The figure shows three views and two pictorial views of one solid part (mm, origin at its lowest corner). Answer the questions. Round coordinates to 2 decimals unless told otherwise and drop trailing zeros. Order: outer loops, then holes, each group sorted by start corner. A loop starts at its lowest first (then second) coordinate and runs counter-clockwise, first axis right, second up. Notation, with made-up numbers: (52.5, 15) -> (59.5, 15) arc R26 ccw to (59.5, 45) -> close; hole circle Ø6 at (-25.75, 88.5). An arc over 180 degrees is marked (long way). Return JSON: item names as keys, results as strings. Group by question number.
(1) The part is cut by section A-A (x = 190.5). Determine the outline of the cut face in (y, z) (1 decimal).
(2) Consider line 1 (X direction, y = 2.15, z = 203.2); line 2 (Z direction, x = 190.5, y = 1); line 3 (Z direction, x = 30.48, y = 1.5). Determine where each line is inside the solid, lowest interval first. Write a range as [from, to].
(3) This flat-tipped pin is pushed along its axis until it touches: pin 1 (4 mm diameter, centred on x = 12.7, z = 50.8, fed in from +Y). Where does it stop, or does it pass through?
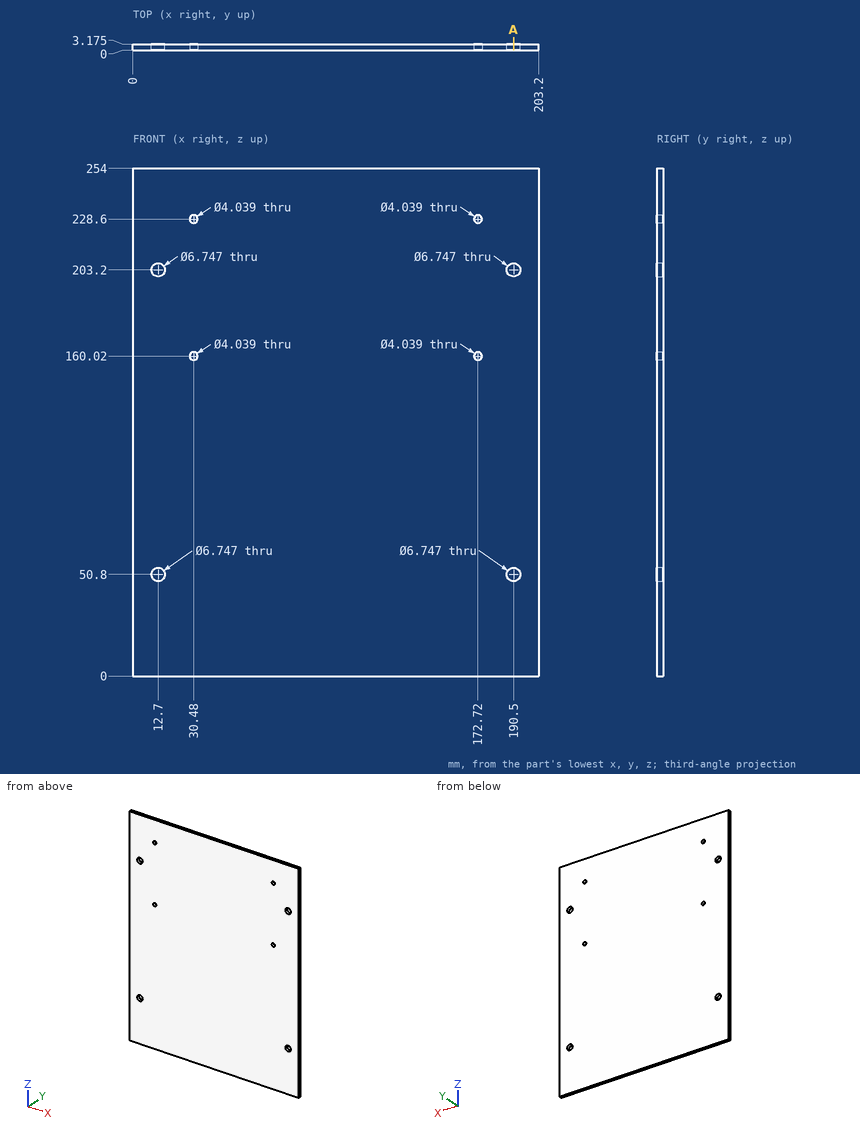
Answer below:
{
 "1": {"outline": "(0, 0) -> (3.2, 0) -> (3.2, 47.4) -> (0, 47.4) -> close; (0, 54.2) -> (3.2, 54.2) -> (3.2, 199.8) -> (0, 199.8) -> close; (0, 206.6) -> (3.2, 206.6) -> (3.2, 254) -> (0, 254) -> close"},
 "2": {"line 1": "x = [0, 9.33], [16.07, 187.13], [193.87, 203.2]", "line 2": "z = [0, 47.43], [54.17, 199.83], [206.57, 254]", "line 3": "z = [0, 158], [162.04, 226.58], [230.62, 254]"},
 "3": {"pin 1": "passes through"}
}
